```python
from build123d import *

# Parameters (mm, degrees)
F0_R     = 2.1717
F1_DEPTH = 9.525
F0_R_2   = 3.429
F2_DEPTH = 3.937
F5_SIZE  = 0.762


with BuildPart() as f1:
    # F0 (on Right) → F1 (new body)
    with BuildSketch(Plane.YZ):
        Circle(F0_R)
    extrude(amount=F1_DEPTH)

    # F0 (on Right) → F2 (join)
    with BuildSketch(Plane.YZ):
        Circle(F0_R_2)
        Circle(F0_R, mode=Mode.SUBTRACT)
        Circle(F0_R)
    extrude(amount=-F2_DEPTH)

    # F3 (on Front) → F4 (revolve, cut)
    with BuildSketch(Plane.XZ):
        with BuildLine():
            Line((6.35, 2.1717), (0, 2.1717))
            ThreePointArc((0, 2.1717), (0.185987, 1.722687), (0.635, 1.5367))
            Line((0.635, 1.5367), (5.715, 1.5367))
            ThreePointArc((5.715, 1.5367), (6.164013, 1.722687), (6.35, 2.1717))
        make_face()
    revolve(axis=Axis((3.39265, 0, 0), (1, 0, 0)), mode=Mode.SUBTRACT)

    # F5
    f5_edges = [f1.edges().sort_by_distance(p)[0] for p in [
        (9.525, -2.1717, 0),
    ]]
    chamfer(f5_edges, length=F5_SIZE)

    # F6 (on Front) → F7 (revolve, cut)
    with BuildSketch(Plane.XZ):
        with BuildLine():
            Line((-1.113861, 3.429), (-3.937, 3.429))
            Line((-3.937, 3.429), (-3.937, 0))
            Line((-3.937, 0), (-3.9116, 0))
            ThreePointArc((-3.9116, 0), (-3.795592, 0.58321), (-3.465231, 1.077631))
            Line((-3.465231, 1.077631), (-1.113861, 3.429))
        make_face()
    revolve(axis=Axis((-3.9243, 0, 0), (1, 0, 0)), mode=Mode.SUBTRACT)


solid = f1.part
```
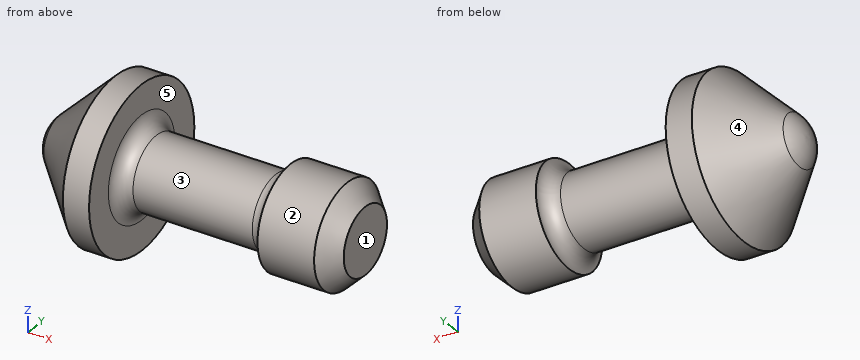
Verification items for the finished model (mm, model axes). Face numbers are marked on the shaded views. A direction names the side the tool comes from. Give positions to 0.01 mm unless a question says otherwise; leave off trailing zeros. Loops run counter-clockwise (first coordinate to the right, second up) from the corner with the lowest first, then second, coordinate; pieces in that order, holes last.
1. Go/stop test with flat-tipped pins: pin 1 Ø2 at (x, z) = (0.5, -1.5) entering from -Y; pin 2 Ø3 at (x, y) = (2.5, 2) entering from -Z. Record where each tip stops, or that it passes through.
2. Section check A-A, the plane x = -0.5. Enter the section's corners in (y, z).
3. Mould release check, pull along X, two halves, no side actions. Record for the marked faces 3, 4 and 5: released by +X, released by -X, zero draft, split by the parting line, or undercut.
4. Section check B-B, the plane x = 4.25. Enter the section's corners in (y, z).
5. Set-up check for the marked faces 1 and 2: record each of +Z, -Z, +X, -X, +Y, -Y from which the full face is reachable in a straight line by a thin tool's end or side.
6. Thickness scan on line 1 (X direction, y = 1, z = -0.5) (3 decimals); line 2 (X direction, y = -0.75, z = -1.5); line 3 (X direction, y = 2.25, z = 2.25). Record the ranges inside material, lowest first.
Geometry says:
1. pin 1: stops at y = -3.37
1. pin 2: stops at z = -1.45
2. outline: circle Ø6.86 at (0, 0)
3. face 3: undercut
3. face 4: released by -X
3. face 5: released by +X
4. outline: circle Ø3.07 at (0, 0)
5. face 1: +Z, -Z, +X, +Y, -Y
5. face 2: +X
6. line 1: x = -3.425 to 9.525
6. line 2: x = -2.87 to 0.24, 6.11 to 9.26
6. line 3: x = -1.36 to 0
